Read the model definition and answer for the solid it produces. Units are mm, in the model's axes. Coordinates: 2 decimals unless noted, no trailing zeros. Order: outer loops, then holes, each group sorted by start corner. A loop starts at its lowest first (then second) coordinate and runs counter-clockwise, first axis right, second up. Notation, with made-up numbers: (-9, -31.5) -> (9, -31.5) arc R24 ccw to (9, 0.5) -> close; hole circle Ø2 at (88, 64.25). An arc over 180 degrees is marked (long way). Answer as a JSON object with one key per item and string values. Group by question number.
1) Section B-B on y = -28 is taken. Determine the outline of the cut face in (x, z), and give its area (3 significant figures).
2) Consider L1, parallel to X at y = 9, z = 1.4; L2, parallel to Y at x = -21, z = 2; L3, parallel to X at y = -6, z = 1.55. Determine where each line is inside the solid, lowest interval first.
3) Section A-A on x = -17 is taken. Determine the outline of the cut face in (y, z), and give its area (3 significant figures).
4) Given pin 1 (1.5 mm diameter, centred on x = 25, z = 2, fed in from -Y), flat-ended and moving along its own axis, determine where the tip first touches the part or whether it passes through.
5) Section C-C on x = 24 is taken. Determine the outline of the cut face in (y, z).
6) Section D-D on z = 1.65 is taken. Count the separate pieces of the cut face and the enclosed holes in it, and give its area (3 significant figures).
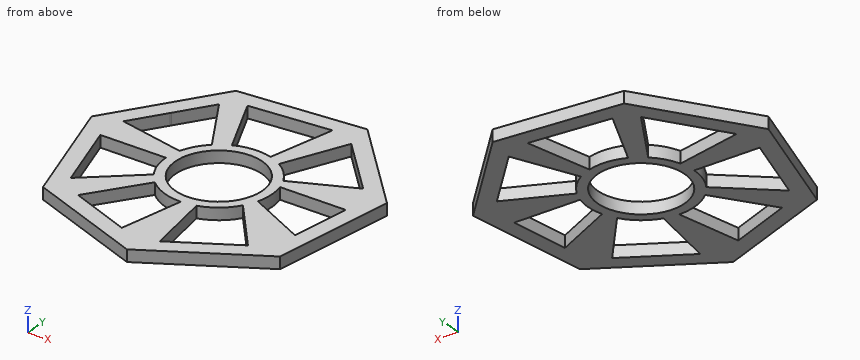
from build123d import *

# Parameters (mm, degrees)
F0_R     = 11
F1_DEPTH = 3


with BuildPart() as f1:
    # F0 (on Top) → F1 (new body)
    with BuildSketch(Plane.XY):
        Polygon((2.837694, -36.586455), (30.374383, -20.59339), (35.037605, 10.907431), (13.317207, 34.194158), (-18.431472, 31.732385), (-36.30111, 5.374778), (-26.83544, -25.029966), align=None)
        with BuildLine():
            Line((-18.923725, -23.596064), (-9.207349, -9.872929))
            ThreePointArc((-9.207349, -9.872929), (-4.948002, -12.560544), (0, -13.5))
            Line((0, -13.5), (-3.394976, -29.72536))
            Line((-3.394976, -29.72536), (-18.923725, -23.596064))
        make_face(mode=Mode.SUBTRACT)
        with BuildLine():
            Line((-24.433495, -18.516342), (-30.198042, 0))
            Line((-30.198042, 0), (-13.5, 0))
            ThreePointArc((-13.5, 0), (-12.954259, -3.799627), (-11.361161, -7.292052))
            Line((-11.361161, -7.292052), (-24.433495, -18.516342))
        make_face(mode=Mode.SUBTRACT)
        with BuildLine():
            Line((22.20563, -20.59339), (6.35273, -29.800614))
            Line((6.35273, -29.800614), (3.645024, -12.998608))
            ThreePointArc((3.645024, -12.998608), (8.03763, -10.846498), (11.37502, -7.270413))
            Line((11.37502, -7.270413), (22.20563, -20.59339))
        make_face(mode=Mode.SUBTRACT)
        with BuildLine():
            Line((29.802458, 3.559528), (27.591791, -11.373886))
            Line((27.591791, -11.373886), (12.876009, -4.056895))
            ThreePointArc((12.876009, -4.056895), (13.497511, -0.259214), (13.022279, 3.559528))
            Line((13.022279, 3.559528), (29.802458, 3.559528))
        make_face(mode=Mode.SUBTRACT)
        with BuildLine():
            Line((-23.782364, 16.302376), (-17.888175, 24.996269))
            Line((-17.888175, 24.996269), (-9.005221, 10.057634))
            ThreePointArc((-9.005221, 10.057634), (-11.35498, 7.301672), (-12.887512, 4.020203))
            Line((-12.887512, 4.020203), (-29.721297, 7.542486))
            Line((-29.721297, 7.542486), (-23.948342, 16.057559))
            Line((-23.948342, 16.057559), (-23.782364, 16.302376))
        make_face(mode=Mode.SUBTRACT)
        with BuildLine():
            Line((-12.75861, 27.945212), (7.703053, 29.626006))
            Line((7.703053, 29.626006), (3.895945, 12.925618))
            ThreePointArc((3.895945, 12.925618), (-0.85982, 13.472591), (-5.507469, 12.325493))
            Line((-5.507469, 12.325493), (-12.75861, 27.945212))
        make_face(mode=Mode.SUBTRACT)
        Circle(F0_R, mode=Mode.SUBTRACT)
        with BuildLine():
            Line((14.222467, 27.209421), (27.425496, 13.054278))
            Line((27.425496, 13.054278), (12.024924, 6.136058))
            ThreePointArc((12.024924, 6.136058), (9.926723, 9.149326), (7.094178, 11.485758))
            Line((7.094178, 11.485758), (14.222467, 27.209421))
        make_face(mode=Mode.SUBTRACT)
    extrude(amount=F1_DEPTH)


solid = f1.part
Worked answers:
{
 "1": {"outline": "(-19.21, 0) -> (-7.77, 0) -> (-7.77, 3) -> (-19.21, 3) -> close; (-3.03, 0) -> (6.06, 0) -> (6.06, 3) -> (-3.03, 3) -> close; (9.45, 0) -> (17.62, 0) -> (17.62, 3) -> (9.45, 3) -> close", "area": "86.1 mm²"},
 "2": {"L1": "x = -33.84 to -28.73, -10.06 to -6.32, 6.32 to 10.06, 18.4 to 34.76", "L2": "y = -27.3 to -15.57, 0 to 5.72, 20.41 to 27.94", "L3": "x = -32.76 to -28.33, -12.09 to -9.22, 9.22 to 16.78, 28.39 to 32.53"},
 "3": {"outline": "(-28.86, 0) -> (-24.36, 0) -> (-24.36, 3) -> (-28.86, 3) -> close; (-20.88, 0) -> (-12.13, 0) -> (-12.13, 3) -> (-20.88, 3) -> close; (0, 0) -> (4.88, 0) -> (4.88, 3) -> (0, 3) -> close; (23.5, 0) -> (31.84, 0) -> (31.84, 3) -> (23.5, 3) -> close", "area": "79.4 mm²"},
 "4": {"pin 1": "stops at y = -24.15"},
 "5": {"outline": "(-24.3, 0) -> (-9.59, 0) -> (-9.59, 3) -> (-24.3, 3) -> close; (3.56, 0) -> (11.52, 0) -> (11.52, 3) -> (3.56, 3) -> close; (16.73, 0) -> (22.74, 0) -> (22.74, 3) -> (16.73, 3) -> close"},
 "6": {"separate pieces": "1", "enclosed holes": "8", "area": "1,810 mm²"}
}
